Read the model definition and answer for the solid it produces. Units are mm, in the model's axes. A direction names the side the tool comes from. Coordinates: 2 decimals unless noted, no trailing zeros. Loops run counter-clockwise (first coordinate to the right, second up) from the corner with the lowest first, then second, coordinate; pieces in that order, holes last. Notation, with made-up numbers: M 44,62.25 L 82,62.25 A8 ccw 82,72.25 Z; hole C -5.75,-15 d1. An arc over 180 degrees is marked long. Use one line per item in the form item = value. Start each with the question number.
1. The part is cut by section B-B (x = 17.5). Give the vertices of the cut face in (y, z), plus the area to 3 significant figures.
2. Find the intervals of material crossed by probe 1 along X at (y, z) = (3.75, 0); probe 2 along X at (y, z) = (7.65, 0); probe 3 along Y at (x, z) = (10, -2), in increasing order. Write a range as [from, to].
3. For a pull along Z with two mould halves and no side action, classify faces 4 (the flat face through (12, 2.286, -3)), 5 (the cylindrical face through (-20.44, 1.16, -4.54)), 6 (the flat face through (2.54, 1, 0)) as released by +Z, released by -Z, zero draft, split by the parting line, or undercut.
4. Flat-ended cylindrical pins translate along their axes: pin 1 (0.7 mm diameter, centred on y = 1.5, z = 0.5, fed in from -X); pin 2 (3 mm diameter, centred on y = 2, z = -4, fed in from +X); pin 3 (4 mm diameter, centred on x = -16.002, z = 0, fed in from -Y); pin 4 (4 mm diameter, centred on x = 17.5, z = -1, fed in from +Y). Find the tip coordinate at first contact, or state that the pin passes through.
5. The part is cut by section A-A (y = 4.25). Give the vertices of the cut face in (x, z) (3 decimals), plus the area to 3 significant figures.
6. A tool of negligible diameter and unlimited length cuts with its end or side. For faces 1 (the cylindrical face through (-12.283, 5.103, -1.542)), 2 (the flat face through (27.94, 1, 0)), 3 (the cylindrical face through (37.023, 0.388, 0.131)), from which of +Z, -Z, +X, -X, +Y, -Y can it reach the whole face along a straight path? Write none if from no direction.
7. The part is cut by section C-C (z = 5.25). Give the vertices of the cut face in (x, y).
Autodesk Inventor part; units mm, degrees
ref_plane "YZ Plane" through (0, 0, 0) normal (1, 0, 0) x (0, 1, 0)
ref_plane "XZ Plane" through (0, 0, 0) normal (0, 1, 0) x (-1, 0, 0)
ref_plane "XY Plane" through (0, 0, 0) normal (0, 0, 1) x (1, 0, 0)
sketch "Sketch1" plane through (0, 0, 0) normal (0, 1, 0) x (-1, 0, 0)
  line L0 (22.352, 6.35) -> (-46.355, 6.35)
  line L1 (-46.355, 6.35) -> (-46.355, -6.35)
  line L2 (-46.355, -6.35) -> (22.352, -6.35)
  line L3 (22.352, -6.35) -> (22.352, 6.35)
  line L4 (-2.54, -2.54) -> (2.54, -2.54)
  line L5 (2.54, -2.54) -> (2.54, 2.54)
  line L6 (2.54, 2.54) -> (-2.54, 2.54)
  line L7 (-2.54, 2.54) -> (-2.54, -2.54)
  line L8 (-2.54, -2.54) -> (2.54, 2.54) construction
  line L9 (2.54, -2.54) -> (-2.54, 2.54) construction
  line L10 (-10.16, 2.54) -> (-15.24, 2.54)
  line L11 (-15.24, 2.54) -> (-15.24, -2.54)
  line L12 (-15.24, -2.54) -> (-10.16, -2.54)
  line L13 (-10.16, -2.54) -> (-10.16, 2.54)
  line L14 (-10.16, 2.54) -> (-15.24, -2.54) construction
  line L15 (-15.24, 2.54) -> (-10.16, -2.54) construction
  line L16 (-22.86, 2.54) -> (-27.94, 2.54)
  line L17 (-27.94, 2.54) -> (-27.94, -2.54)
  line L18 (-27.94, -2.54) -> (-22.86, -2.54)
  line L19 (-22.86, -2.54) -> (-22.86, 2.54)
  line L20 (-22.86, 2.54) -> (-27.94, -2.54) construction
  line L21 (-27.94, 2.54) -> (-22.86, -2.54) construction
  point P0 (0, 0)
  point P1 (-12.7, 0)
  point P2 (-25.4, 0)
  dimension "d0" = 68.707
  dimension "d1" = 12.7
  dimension "d2" = 5.08
  dimension "d3" = 5.08
  dimension "d4" = 5.08
  dimension "d5" = 5.08
  dimension "d6" = 12.7
  dimension "d7" = 12.7
  dimension "d8" = 6.35
  dimension "d9" = 22.352
  dimension "d37" = 5.08
  dimension "d38" = 5.08
extrude "Extrusion1" add sketch "Sketch1" along normal blind 2.286
sketch "Sketch2" plane through (0, 2.286, 0) normal (0, 1, 0) x (1, 0, 0)
  line L0 (-22.352, 6.35) -> (-22.352, -6.35)
  circle A0 centre (-16.002, 0) radius 4.0259
  point P0 (0, 0)
  dimension "d12" = 6.35
  dimension "d13" = 8.0518
extrude "Extrusion2" add sketch "Sketch2" along normal blind 5.715
sketch "Sketch3" plane through (-16.002, 8.001, 0) normal (0, 1, 0) x (1, 0, 0)
  circle A0 centre (0, 0) radius 2.9845
  point P0 (16.002, 0)
  dimension "d16" = 5.969
extrude "Extrusion3" cut sketch "Sketch3" against normal blind 0.7874
sketch "Sketch4" plane through (0, 0, 0) normal (0, -1, 0) x (1, 0, 0)
  circle A0 centre (-16.002, 0) radius 2.9845
  circle A1 centre (-16.002, 0) radius 2.9845
  point P0 (0, 0)
  dimension "d39" = 5.969
extrude "Extrusion4" cut sketch "Sketch4" against normal blind 0.7874
sketch "Sketch5" plane through (-16.002, 7.2136, 0) normal (0, 1, 0) x (1, 0, 0)
  circle A0 centre (0, 0) radius 2.5781
  point P0 (16.002, 0)
  dimension "d21" = 5.1562
extrude "Extrusion5" cut sketch "Sketch5" against normal through all
sketch "Sketch6" plane through (0, 2.286, 0) normal (0, 1, 0) x (1, 0, 0)
  line L0 (46.355, -6.35) -> (46.355, 6.35)
  circle A0 centre (40.005, 0) radius 4.0259
  point P0 (0, 0)
  dimension "d24" = 6.35
  dimension "d25" = 8.0518
extrude "Extrusion6" add sketch "Sketch6" along normal blind 5.715
sketch "Sketch7" plane through (40.005, 8.001, 0) normal (0, 1, 0) x (1, 0, 0)
  circle A0 centre (0, 0) radius 2.9845
  point P0 (-40.005, 0)
  dimension "d28" = 5.969
extrude "Extrusion7" cut sketch "Sketch7" against normal blind 0.7874
sketch "Sketch8" plane through (0, 0, 0) normal (0, -1, 0) x (1, 0, 0)
  circle A0 centre (40.005, 0) radius 2.9845
  circle A1 centre (40.005, 0) radius 2.9845
  point P0 (0, 0)
  dimension "d40" = 5.969
extrude "Extrusion8" cut sketch "Sketch8" against normal blind 0.7874
sketch "Sketch9" plane through (40.005, 7.2136, 0) normal (0, 1, 0) x (1, 0, 0)
  circle A0 centre (0, 0) radius 2.5781
  point P0 (-40.005, 0)
  dimension "d33" = 5.1562
extrude "Extrusion9" cut sketch "Sketch9" against normal through all
fillet "Fillet1" radius 6.35 4 edges at (46.355, 1.143, 6.35) (46.355, 1.143, -6.35) (-22.352, 1.143, 6.35) (-22.352, 1.143, -6.35)
sketch "Sketch12" plane through (-16.002, 8.001, 0) normal (0, 1, 0) x (1, 0, 0)
  circle A0 centre (0, 0) radius 4.0259
  line L0 (0, 0) -> (4.0259, 0) construction
  line L1 (0, 0) -> (4.0259, 0) construction
  circle A1 centre (0, 0) radius 2.9845
  line L2 (-2.9392, 0.5183) -> (-3.9647, 0.6991)
  line L3 (-2.9392, -0.5183) -> (-3.9647, -0.6991)
  arc A2 (-2.9392, 0.5183) -> (-2.9392, -0.5183) centre (0, 0) ccw
  arc A3 (-3.9647, 0.6991) -> (-3.9647, -0.6991) centre (0, 0) ccw
  point P0 (16.002, 0)
  point P1 (-2.9392, 0.5183)
extrude "Extrusion11" cut sketch "Sketch12" against normal blind 0.762 contours L2 A1 L3 A0 picked at (-3.6725, 0.0578)
properties part number "VexLegoMountThick"
Computed values:
q1.outline = M 0,-6.35 L 2.29,-6.35 L 2.29,6.35 L 0,6.35 Z
q1.area = 29.0 mm²
q2.probe_1 = [-20.03, -18.58], [-13.42, -11.98], [35.98, 37.43], [42.58, 44.03]
q2.probe_2 = [-13.02, -11.98], [35.98, 37.02], [42.99, 44.03]
q2.probe_3 = [0, 2.29]
q3.face_4 = zero draft
q3.face_5 = released by -Z
q3.face_6 = undercut
q4.pin_1 = -22.35
q4.pin_2 = 45.84
q4.pin_3 = through
q4.pin_4 = 2.29
q5.outline = C -16.002,0 d8.052; C 40.005,0 d8.052; hole C -16.002,0 d5.156; hole C 40.005,0 d5.156
q5.area = 60.1 mm²
q6.face_1 = +Y
q6.face_2 = +Y, -Y
q6.face_3 = -Y
q7.outline = M -19.57,0 L 43.58,0 L 43.58,2.29 L -19.57,2.29 Z
